Can you work these out from the model? Positions are in its coordinate system, mm. A direction names the side the tool comes from. Give positions to 0.01 mm unless a question says otherwise; leave off trailing zeros. Loops run counter-clockwise (first coordinate to the right, second up) from the corner with the lowest first, then second, coordinate; pieces in that order, holes last. Notation, with made-up numbers: M 13.5,-28.75 L 61.5,-28.75 A26 cw 61.5,4.25 Z; hole C -33.5,-26 d6. An arc over 180 degrees is marked long. Put each result on its own line as item: value. Start each with the question number.
1) Please list where these lines run through material, in increasing order: line 1 along Z through (x, y) = (30, 19.5); line 2 along Z through (x, y) = (98, 83); line 3 along Y through (x, z) = (89.5, 11.25). Write a range as from..to.
2) Imagine slicing it at C-C (y = 85). Write out the boundary of the cut face in (x, z), then the cut area to 3 significant figures.
3) If we mould it in two halves opening along Y, with no side actions, what happens to faces 1 (the flat face through (69.79, 24.84, 11.92)), 2 (the flat face through (180, 83, 3)), 3 (the flat face through (114.653, 85.229, 13.07))? For each: +Y half, -Y half, draft (parallel to the pull), parting line (faces both ways), or undercut.
4) For P1, Ø4, axis at x = 160, y = 143.5, coming from the +Z side; P2, Ø1, axis at y = 117.5, z = 12, coming from the -X side; P3, Ø1, axis at x = 141, y = 55.5, coming from the -Z side; P4, Ø6, axis at y = 146, z = 14.5, coming from the -X side, each with a flat end and sliding along its axis, tell me the tip position at first contact or that it passes through.
5) Imagine slicing it at A-A (z = 16). Write out the boundary of the cut face in (x, y).
6) Imagine slicing it at D-D (x = 26). Write out the boundary of the cut face in (y, z), then the cut area to 3 significant figures.
7) Imagine slicing it at B-B (x = 159). Write out the boundary of the cut face in (y, z).
8) For faces 4 (the flat face through (28.167, 82.79, 11.916)), 5 (the flat face through (163.3, 62.61, 11.92)), 6 (the cylindrical face through (138.4, 25.55, 11.92)), 7 (the flat face through (81, 77, 2)), which set-ups out of +Z, -Z, +X, -X, +Y, -Y let a thin tool reach every point of the face, with its end or its side?
from build123d import *

# Parameters (mm, degrees)
PAD_DEPTH       = 6
PAD001_DEPTH    = 12
POCKET_DEPTH    = 10
SKETCH003_R     = 13.5
POCKET001_DEPTH = 6


with BuildPart() as part:
    # Sketch → Pad (new body)
    with BuildSketch(Plane.XY):
        with BuildLine():
            ThreePointArc((2, 166), (0.585786, 165.414214), (0, 164))
            Line((0, 4.242641), (0, 164))
            Line((0, 4.242641), (4.242641, 0))
            Line((178, 0), (4.242641, 0))
            ThreePointArc((178, 0), (179.414214, 0.585786), (180, 2))
            Line((180, 161.757359), (180, 2))
            Line((175.757359, 166), (180, 161.757359))
            Line((175.757359, 166), (2, 166))
        make_face()
    extrude(amount=PAD_DEPTH)

    # Sketch001 (on Face10 of Pad) → Pad001 (join)
    with BuildSketch(Plane.XY.offset(6)):
        with BuildLine():
            ThreePointArc((56.618237, 141.695686), (35.433188, 152.851689), (35.337576, 128.908975))
            ThreePointArc((38.028145, 122.339284), (37.758773, 126.064762), (35.337576, 128.908975))
            Line((38.028145, 122.339284), (18.026388, 42.116616))
            Line((18.026388, 42.116616), (21.116616, 36.973612))
            Line((21.116616, 36.973612), (119.851347, 12.356279))
            ThreePointArc((119.851347, 12.356279), (129.691827, 13.826948), (135.610177, 21.825139))
            ThreePointArc((142.883482, 26.195382), (138.341722, 25.516611), (135.610177, 21.825139))
            Line((142.883482, 26.195382), (149.78317, 24.475096))
            Line((149.78317, 24.475096), (154.49759, 27.307806))
            Line((171.860307, 96.945859), (154.49759, 27.307806))
            ThreePointArc((171.860307, 96.945859), (171.519805, 100.83781), (168.855362, 103.695076))
            Line((151.638909, 112.849226), (168.855362, 103.695076))
            ThreePointArc((151.638909, 112.849226), (148.639111, 114.216313), (145.495068, 115.207626))
            Line((61.155784, 136.235771), (145.495068, 115.207626))
            ThreePointArc((56.618237, 141.695686), (57.992845, 138.222619), (61.155784, 136.235771))
        make_face()
    extrude(amount=PAD001_DEPTH)

    # Sketch002 (on Face26 of Pad001) → Pocket (cut)
    with BuildSketch(Plane.XY.offset(18)):
        with BuildLine():
            ThreePointArc((44.26968, 90.573005), (43.039189, 89.66249), (42.812933, 88.14857))
            Line((42.812933, 88.14857), (52.73173, 48.366445))
            ThreePointArc((52.73173, 48.366445), (53.642246, 47.135954), (55.156166, 46.909698))
            Line((55.156166, 46.909698), (118.225388, 62.634621))
            ThreePointArc((118.225388, 62.634621), (119.455879, 63.545136), (119.682135, 65.059056))
            Line((109.763338, 104.841181), (119.682135, 65.059056))
            ThreePointArc((109.763338, 104.841181), (108.852822, 106.071672), (107.338902, 106.297928))
            Line((107.338902, 106.297928), (44.26968, 90.573005))
        make_face()
    extrude(amount=-POCKET_DEPTH, mode=Mode.SUBTRACT)

    # Sketch003 (on Face35 of Pocket) → Pocket001 (cut)
    with BuildSketch(Plane.XY.offset(8)):
        with Locations((81.247534, 76.603813)):
            Circle(SKETCH003_R)
    extrude(amount=-POCKET001_DEPTH, mode=Mode.SUBTRACT)


solid = part.part
Recorded:
1. line 1: 0..6
1. line 2: 0..8
1. line 3: 19.92..55.47, 101.85..129.17
2. outline: M 0,0 L 180,0 L 180,6 L 168.88,6 L 168.88,18 L 114.71,18 L 114.71,8 L 91.82,8 L 91.82,2 L 70.68,2 L 70.68,8 L 43.6,8 L 43.6,18 L 28.72,18 L 28.72,6 L 0,6 Z
2. area: 1,920 mm²
3. face 1: -Y half
3. face 2: draft
3. face 3: undercut
4. P1: z = 6
4. P2: x = 36.7
4. P3: z = 0
4. P4: x = 28.81
5. outline: M 18.03,42.12 L 21.12,36.97 L 119.85,12.36 A13 ccw 135.61,21.83 A6 cw 142.88,26.2 L 149.78,24.48 L 154.5,27.31 L 171.86,96.95 A6 ccw 168.86,103.7 L 151.64,112.85 A27 ccw 145.5,115.21 L 61.16,136.24 A6 cw 56.62,141.7 A14 ccw long 35.34,128.91 A6 cw 38.03,122.34 Z; hole M 42.81,88.15 L 52.73,48.37 A2 ccw 55.16,46.91 L 118.23,62.63 A2 ccw 119.68,65.06 L 109.76,104.84 A2 ccw 107.34,106.3 L 44.27,90.57 A2 ccw Z
6. outline: M 0,0 L 166,0 L 166,6 L 74.1,6 L 74.1,18 L 35.76,18 L 35.76,6 L 0,6 Z
6. area: 1,460 mm²
7. outline: M 0,0 L 166,0 L 166,6 L 108.94,6 L 108.94,18 L 45.37,18 L 45.37,6 L 0,6 Z
8. face 4: +Z, -X
8. face 5: +Z, +X, -Y
8. face 6: +Z, -Y
8. face 7: +Z
